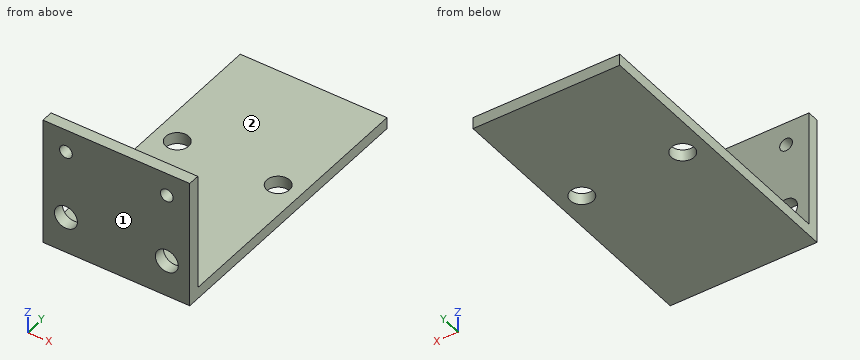
from build123d import *

# Parameters (mm, degrees)
F1_DEPTH = 12.7
F3_R     = 1.985
F3_R_2   = 1.1
F4_DEPTH = 49.211
F2_R     = 1.985
F5_DEPTH = 2.001


with BuildPart() as f1:
    # F0 (on Right) → F1 (new body, symmetric)
    with BuildSketch(Plane.YZ):
        Polygon((-22.605, -9.115), (-22.605, 11.115), (-24.605, 11.115), (-24.605, -11.115), (24.605, -11.115), (24.605, -9.115), align=None)
    extrude(amount=F1_DEPTH, both=True)

    # F3 (on face) → F4 (cut, through all)
    with BuildSketch(Plane.XZ.offset(24.605)):
        with Locations((8.73, -4.765)):
            Circle(F3_R)
        with Locations((8.73, 7.145)):
            Circle(F3_R_2)
        with Locations((-8.73, -4.765)):
            Circle(F3_R)
        with Locations((-8.73, 7.145)):
            Circle(F3_R_2)
    extrude(amount=-F4_DEPTH, mode=Mode.SUBTRACT)

    # F2 (on face) → F5 (cut, through all)
    with BuildSketch(Plane.XY.offset(-9.115)):
        with Locations((-8.73, 3.175)):
            Circle(F2_R)
        with Locations((8.73, 3.175)):
            Circle(F2_R)
    extrude(amount=-F5_DEPTH, mode=Mode.SUBTRACT)


solid = f1.part
For this review, take the finished solid that the model builds, in its own axes (mm). Face numbers are marked on the shaded views. A direction names the side the tool comes from. Round coordinates to 2 decimals unless told otherwise and drop trailing zeros. Loops run counter-clockwise (first coordinate to the right, second up) from the corner with the lowest first, then second, coordinate; pieces in that order, holes last. Notation, with made-up numbers: (15, 7.5) - (69, 7.5) arc R20 cw to (69, 33.5) - close; hole circle Ø11 at (47.5, 9). An arc over 180 degrees is marked (long way). Answer as CSV lines item,"result".
(1) Consider section D-D on y = 20. Give the boundary of the cut face in (x, z) (3 decimals), then the cut area to 3 significant figures.
Checked values:
outline,"(-12.7, -11.115) - (12.7, -11.115) - (12.7, -9.115) - (-12.7, -9.115) - close"
area,"50.8 mm2"
(2) Wall thickness on line 1 (Z direction, x = -8.73, y = -24.05) (3 decimals); line 2 (Y direction, x = -8.73, z = -10.05) (3 decimals); line 3 (Z direction, x = -1, y = 5) (3 decimals): over which ranges is each line inside the solid? List them lowest first.
Checked values:
line 1,"z = -11.115 to -6.75, -2.78 to 6.045, 8.245 to 11.115"
line 2,"y = -24.605 to 1.19, 5.16 to 24.605"
line 3,"z = -11.115 to -9.115"
(3) Consider section B-B on x = 1.5. Give the boundary of the cut face in (y, z) (3 decimals).
Checked values:
outline,"(-24.605, -11.115) - (24.605, -11.115) - (24.605, -9.115) - (-22.605, -9.115) - (-22.605, 11.115) - (-24.605, 11.115) - close"
(4) Consider section C-C on z = 3.5. Give the boundary of the cut face in (x, y) (3 decimals).
Checked values:
outline,"(-12.7, -24.605) - (12.7, -24.605) - (12.7, -22.605) - (-12.7, -22.605) - close"
(5) Tool access review of the marked faces 1 and 2: name each direction out of +Z, -Z, +X, -X, +Y, -Y from which nothing blocks a thin tool from reaching the whole face with its end or side.
Checked values:
face 1,"+Z, -Z, +X, -X, -Y"
face 2,"+Z, +X, -X, +Y"
(6) Consider section A-A on x = -8.73. Give the boundary of the cut face in (y, z) (3 decimals).
Checked values:
outline,"(-24.605, -11.115) - (1.19, -11.115) - (1.19, -9.115) - (-22.605, -9.115) - (-22.605, -6.75) - (-24.605, -6.75) - close; (-24.605, -2.78) - (-22.605, -2.78) - (-22.605, 6.045) - (-24.605, 6.045) - close; (-24.605, 8.245) - (-22.605, 8.245) - (-22.605, 11.115) - (-24.605, 11.115) - close; (5.16, -11.115) - (24.605, -11.115) - (24.605, -9.115) - (5.16, -9.115) - close"
(7) Insertion check: P1, Ø4.5, axis at x = -8.73, z = -4.765, coming from the +Y side (3 decimals); P2, Ø7.5, axis at x = -2, y = -9.5, coming from the +Z side (3 decimals); P3, Ø1.3, axis at x = -8.73, z = 7.145, coming from the +Y side. Each pin has a flat end and moves straight along its axis. Give the tip position at first contact, or say it passes through.
Checked values:
P1,"stops at y = -22.605"
P2,"stops at z = -9.115"
P3,"passes through"
